```python
from build123d import *

# Parameters (mm, degrees)
F0_W     = 19.05
F0_H     = 19.05
F0_W_2   = 15.875
F0_H_2   = 15.875
F1_DEPTH = 107.95
F2_R     = 1.5875
F3_R     = 1.5875
F4_R     = 3.2385
F4_R_2   = 2.5796875
F5_DEPTH = 19.05
F6_DEPTH = 3.175


# Not quite as in the source:
# - a length typed as a fraction of an inch, garbled in the dataset ("3 / 203.2 mm" for 3/8 in), is restored


with BuildPart() as f1:
    # F0 (on Front) → F1 (new body, symmetric)
    with BuildSketch(Plane.XZ):
        Rectangle(F0_W, F0_H)
        with Locations((-0.0127, 0)):
            Rectangle(F0_W_2, F0_H_2, mode=Mode.SUBTRACT)
    extrude(amount=F1_DEPTH, both=True)

    # F2
    f2_edges = [f1.edges().sort_by_distance(p)[0] for p in [
        (-9.525, 0, 9.525),
        (-9.525, 0, -9.525),
        (9.525, 0, -9.525),
        (9.525, 0, 9.525),
    ]]
    fillet(f2_edges, radius=F2_R)

    # F3
    f3_edges = [f1.edges().sort_by_distance(p)[0] for p in [
        (-7.9502, 0, 7.9375),
        (-7.9502, 0, -7.9375),
        (7.9248, 0, 7.9375),
        (7.9248, 0, -7.9375),
    ]]
    fillet(f3_edges, radius=F3_R)

    # F4 (on face) → F5 (cut)
    with BuildSketch(Plane(origin=(-9.525, 0, 0), x_dir=(0, -1, 0), z_dir=(-1, 0, 0))):
        with Locations((-103.1875, 0)):
            Circle(F4_R)
        with Locations((63.5, 0)):
            Circle(F4_R_2)
        with Locations((95.25, 0)):
            Circle(F4_R_2)
    extrude(amount=-F5_DEPTH, mode=Mode.SUBTRACT)

    # F6 (cut): a face of the model
    f6_faces = [f1.faces().sort_by_distance(p)[0] for p in [
        (-8.2196076836, -107.95, 0),
    ]]
    extrude(f6_faces, amount=-F6_DEPTH, mode=Mode.SUBTRACT)


solid = f1.part
```
Source: CAD feature listing. Evaluate the final solid. Frame: model axes, mm. A direction names the side the tool comes from. Round coordinates to 2 decimals unless told otherwise and drop trailing zeros.
(1) Material intervals for probe 1 along Y at (x, z) = (8.75, -0.25) (3 decimals); probe 2 along Z at (x, y) = (1, -52) (1 decimal); probe 3 along X at (y, z) = (42.5, 2) (3 decimals), sorted ascending.
From the geometry:
probe 1: y = -104.775 to -97.818, -92.682 to -66.068, -60.932 to 99.959, 106.416 to 107.95
probe 2: z = -9.5 to -7.9, 7.9 to 9.5
probe 3: x = -9.525 to -7.95, 7.925 to 9.525
(2) Pull-direction query (Z, two-part tool) for faces 1 (the flat face through (0, 0, -9.525)), 2 (the flat face through (-7.95, 0, 0)), 3 (the flat face through (-9, -104.775, 0)), 4 (the flat face through (0, 0, 9.525)); classes: +Z half, -Z half, draft (parallel to the pull), parting line (faces both ways), or undercut.
From the geometry:
face 1: -Z half
face 2: undercut
face 3: draft
face 4: +Z half
(3) Access query for faces 5 (the cylindrical face through (-8.75, -64.69, -2.29)), 6 (the flat face through (7.925, 0, 0)). Directions: +Z, -Z, +X, -X, +Y, -Y. A direction counts if a zero-diameter tool reaches every point of the face in a straight line with its end or side. Return the directions, or none.
From the geometry:
face 5: +X, -X
face 6: +Y, -Y
(4) Section query B-B (z = 0). Give the number of separate pieces and of enclosed holes in the cut face, and give its area (3 significant figures).
From the geometry:
separate pieces: 8
enclosed holes: 0
area: 622 mm2
